The model under review builds one solid part; all positions refer to its coordinate system, in mm. Give positions to 0.01 mm unless a question says otherwise; leave off trailing zeros. Loops run counter-clockwise (first coordinate to the right, second up) from the corner with the lowest first, then second, coordinate; pieces in that order, holes last. Notation, with made-up numbers: M -28.75,-28 L -3.75,-28 A27 cw -3.75,6 Z; hole C 21.5,89 d4. An arc over 180 degrees is marked long. Write item = value, one per line. Start each with the question number.
1. We need section A-A on y = 49.5. Give the boundary of the cut face in (x, z), then the cut area to 3 significant figures.
2. Wall thickness on line 1 along Y through (x, z) = (518.5, -278): over which ranges is the line inside the solid? List them lowest first. Write a range as from..to.
3. We need section B-B on x = 36. Give the boundary of the cut face in (y, z).
4. For pin 1 (12 mm diameter, centred on x = 297, y = 60.5, fed in from +Z); pin 2 (6 mm diameter, centred on x = 516, y = 52.5, fed in from -Z), all flat-tipped, find the tip position at first contact; note any pin that passes through.
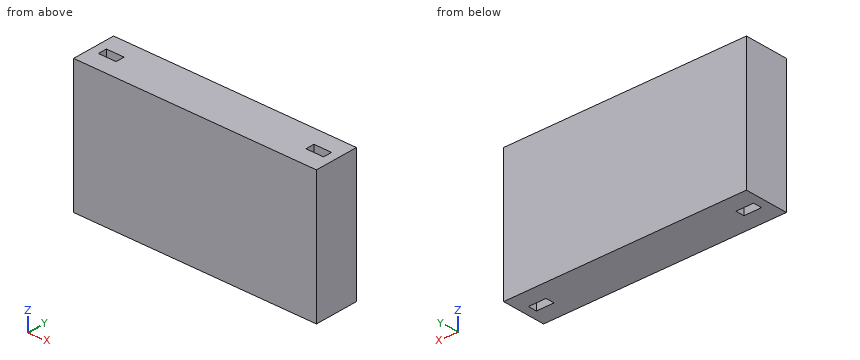
from build123d import *

# Parameters (mm, degrees)
SKETCH1_W           = 300
SKETCH1_H           = 100
BOSS_EXTRUDE1_DEPTH = 550
SKETCH2_W           = 40
SKETCH2_H           = 20
CUT_EXTRUDE1_DEPTH  = 25


with BuildPart() as part:
    # Sketch1 → Boss-Extrude1 (new body)
    with BuildSketch(Plane(origin=(0, 0, 0), x_dir=(0, 0, -1), z_dir=(1, 0, 0))):
        with Locations((150, 50)):
            Rectangle(SKETCH1_W, SKETCH1_H)
    extrude(amount=BOSS_EXTRUDE1_DEPTH)

    # Sketch2 → Cut-Extrude1 (cut)
    with BuildSketch(Plane.XY):
        with Locations((40, 50)):
            Rectangle(SKETCH2_W, SKETCH2_H)
        with Locations((510, 50)):
            Rectangle(SKETCH2_W, SKETCH2_H)
    cut_extrude1 = extrude(amount=-CUT_EXTRUDE1_DEPTH, mode=Mode.SUBTRACT)

    # Mirror1: Cut-Extrude1 across plane
    add(cut_extrude1.mirror(Plane.XY.offset(-150)), mode=Mode.SUBTRACT)


solid = part.part
Final values:
q1.outline = M 0,-300 L 20,-300 L 20,-275 L 60,-275 L 60,-300 L 490,-300 L 490,-275 L 530,-275 L 530,-300 L 550,-300 L 550,0 L 530,0 L 530,-25 L 490,-25 L 490,0 L 60,0 L 60,-25 L 20,-25 L 20,0 L 0,0 Z
q1.area = 161,000 mm²
q2.line_1 = 0..40, 60..100
q3.outline = M 0,-300 L 40,-300 L 40,-275 L 60,-275 L 60,-300 L 100,-300 L 100,0 L 60,0 L 60,-25 L 40,-25 L 40,0 L 0,0 Z
q4.pin_1 = 0
q4.pin_2 = -275
